Geometry: see drawing. Coordinates: mm, zero at the bounding-box minimum. A direction names the side the tool comes from. Give positions to 0.01 mm unless a question says otherwise; leave off trailing zeros. Loops run counter-clockwise (first coordinate to the right, second up) from the corner with the lowest first, then second, coordinate; pieces in that order, holes last. Notation, with made-up numbers: M 87,55.5 L 143,55.5 A28 ccw 143,87.5 Z; hole C 59,-25 d7. An arc over 180 degrees is marked long. Return JSON: item names as keys, results as strings. Group by question number.
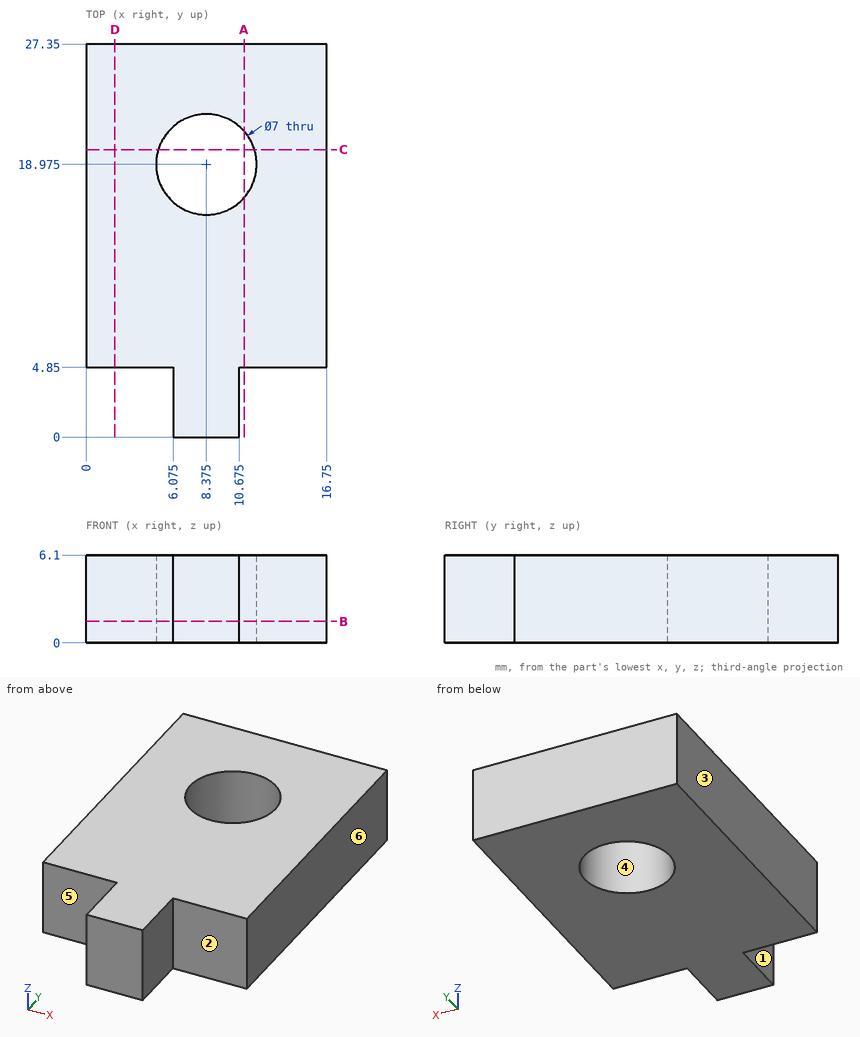
Item 1: First-contact query: pin 1 Ø1 at (x, z) = (15, 3.5) entering from -Y; pin 2 Ø4 at (x, y) = (14, 9.5) entering from -Z. Flat tips, straight axial feed; report the tip coordinate or a pass-through.
Item 2: Reachability of the marked faces 1, 2 and 3 from +Z, -Z, +X, -X, +Y, -Y: full face, straight path, thin tool, end or side. Return the list, or none.
Item 3: Section A-A, the plane x = 11. Return loops of the section in (y, z).
Item 4: Section D-D, the plane x = 2. Return loops of the section in (y, z), then the cut area to 3 significant figures.
Item 5: Pull-direction query (Y, two-part tool) for the marked faces 4, 5 and 6; classes: pulls with the +Y half, pulls with the -Y half, needs draft (parallel to the pull), parting line crosses it, or undercut.
Item 6: Material intervals for line 1 (X direction, y = 3, z = 3) (3 decimals); line 2 (Y direction, x = 14.5, z = 3); line 3 (Y direction, x = 10.25, z = 3.5), sorted ascending. Write a range as from..to.
Item 7: Section C-C, the plane y = 20. Return loops of the section in (x, z), then the cut area to 3 significant figures.
Item 8: Section B-B, the plane z = 1.5. Return loops of the section in (x, y) (3 decimals), then the cut area to 3 significant figures.
Answer below:
{
 "1": {"pin 1": "y = 4.85", "pin 2": "z = 0"},
 "2": {"face 1": "+Z, -Z, -X, -Y", "face 2": "+Z, -Z, +X, -Y", "face 3": "+Z, -Z, -X, +Y, -Y"},
 "3": {"outline": "M 4.85,0 L 16.66,0 L 16.66,6.1 L 4.85,6.1 Z; M 21.29,0 L 27.35,0 L 27.35,6.1 L 21.29,6.1 Z"},
 "4": {"outline": "M 4.85,0 L 27.35,0 L 27.35,6.1 L 4.85,6.1 Z", "area": "137 mm^2"},
 "5": {"face 4": "undercut", "face 5": "pulls with the -Y half", "face 6": "needs draft"},
 "6": {"line 1": "6.075..10.675", "line 2": "4.85..27.35", "line 3": "0..16.02, 21.93..27.35"},
 "7": {"outline": "M 0,0 L 5.03,0 L 5.03,6.1 L 0,6.1 Z; M 11.72,0 L 16.75,0 L 16.75,6.1 L 11.72,6.1 Z", "area": "61.3 mm^2"},
 "8": {"outline": "M 0,4.85 L 6.075,4.85 L 6.075,0 L 10.675,0 L 10.675,4.85 L 16.75,4.85 L 16.75,27.35 L 0,27.35 Z; hole C 8.375,18.975 d7", "area": "361 mm^2"}
}
